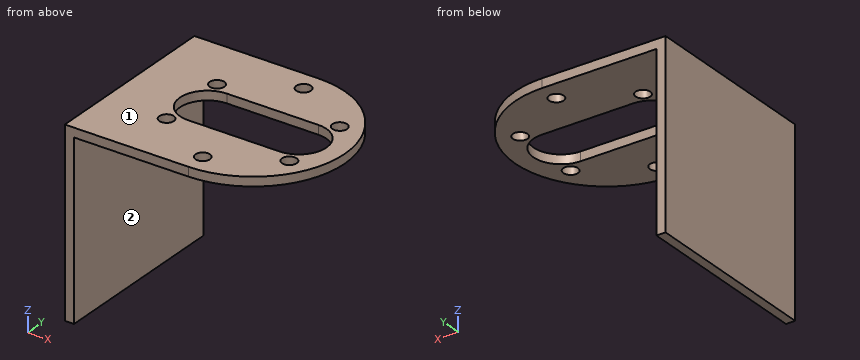
```python
from build123d import *

# Parameters (mm, degrees)
SKETCH_1_W               = 40
SKETCH_1_H               = 40
EXTRUDE_1_DEPTH          = 2
EXTRUDE_2_DEPTH          = 2
SKETCH_3_4_RX            = 1.6
SKETCH_3_4_RY            = 1.6
CUT_EXTRUDE_1_DEPTH      = 2
PATTERN_CIRCULAR_1_COUNT = 6
CUT_EXTRUDE_2_DEPTH      = 65.876806333


with BuildPart() as part:
    # 草图1 → 凸台-拉伸1 (new body)
    with BuildSketch(Plane(origin=(0, 0, 0), x_dir=(0, 0, -1), z_dir=(1, 0, 0))):
        Rectangle(SKETCH_1_W, SKETCH_1_H)
    extrude(amount=EXTRUDE_1_DEPTH)

    # 草图3 → 凸台-拉伸2 (add)
    with BuildSketch(Plane.XY.offset(20)):
        with BuildLine():
            Line((0, 20), (27, 20))
            ThreePointArc((27, 20), (47, 0), (27, -20))
            Line((27, -20), (0, -20))
            Line((0, -20), (0, 20))
        make_face()
    extrude(amount=-EXTRUDE_2_DEPTH)

    # 草图3<4> → 切除-拉伸1 (cut)
    with BuildSketch(Plane.XY.offset(20)):
        with Locations(Location((27.038693052, 15.512584913), (0, 0, 225))):
            Ellipse(SKETCH_3_4_RX, SKETCH_3_4_RY)
    cut_extrude_1 = extrude(amount=-CUT_EXTRUDE_1_DEPTH, mode=Mode.SUBTRACT)

    # 阵列(圆周)1: 切除-拉伸1 ×6 about axis
    pattern_circular_1_axis = Axis((27, 0, 0), (0, 0, 1))
    for i in range(1, PATTERN_CIRCULAR_1_COUNT):
        add(cut_extrude_1.rotate(pattern_circular_1_axis, i * 360 / PATTERN_CIRCULAR_1_COUNT), mode=Mode.SUBTRACT)

    # 草图3<5> → 切除-拉伸2 (cut, through all)
    with BuildSketch(Plane.XY.offset(20)):
        with BuildLine():
            Line((37, -6), (17, -6))
            ThreePointArc((17, -6), (11, 0), (17, 6))
            Line((17, 6), (37, 6))
            ThreePointArc((37, 6), (43, 0), (37, -6))
        make_face()
    extrude(amount=-CUT_EXTRUDE_2_DEPTH, mode=Mode.SUBTRACT)


solid = part.part
```
Read the model definition and answer for the solid it produces. Units are mm, in the model's axes. Face numbers are marked on the shaded views. A direction names the side the tool comes from. Give positions to 0.01 mm unless a question says otherwise; leave off trailing zeros. Write each loop counter-clockwise with the first axis right and the second up, starting at its lowest first coordinate (ties: lowest second). Pieces come first, ordered by that corner, then holes. Notation, with made-up numbers: M 51.5,4.25 L 110.5,4.25 A14 ccw 110.5,17.25 Z; hole C 43,81.5 d4. An arc over 180 degrees is marked long. Put each result on its own line as item: value. Start each with the question number.
1. Which of the six approach directions +Z, -Z, +X, -X, +Y, -Y give full straight-line access (tool end or side, diameter ignored) to the marked faces 1 and 2?
2. The part is cut by section A-A, the plane x = 22.5. Give the vertices of the cut face in (y, z), and give its area (3 significant figures).
3. The part is cut by section C-C, the plane z = 14. Give the vertices of the cut face in (x, y), and give its area (3 significant figures).
4. Each of these flat-tipped pins is pushed along its axis until it touches: pin 1 Ø1 at (x, z) = (31, 19.5) entering from +Y; pin 2 Ø10 at (x, y) = (38.5, 9) entering from -Z; pin 3 Ø11.5 at (y, z) = (-2, -1) entering from +X. Where does it stop, or does it pass through?
5. The part is cut by section B-B, the plane y = 0. Give the vertices of the cut face in (x, z), and give its area (3 significant figures).
6. The part is cut by section D-D, the plane x = 33. Give the vertices of the cut face in (y, z), and give its area (3 significant figures).
7. Consider line 1 along Z through (x, y) = (13, -11); line 2 along X through (y, z) = (15, 12). Determine where each line is inside the solid, lowest interval first.
Final values:
1. face 1: +Z, +X, -X, +Y, -Y
1. face 2: -Z, +X, +Y, -Y
2. outline: M -20,18 L -6,18 L -6,20 L -20,20 Z; M 6,18 L 20,18 L 20,20 L 6,20 Z
2. area: 56.0 mm²
3. outline: M 0,-20 L 2,-20 L 2,20 L 0,20 Z
3. area: 80.0 mm²
4. pin 1: stops at y = 19.69
4. pin 2: stops at z = 18
4. pin 3: stops at x = 2
5. outline: M 0,-20 L 2,-20 L 2,18 L 11,18 L 11,20 L 0,20 Z; M 43,18 L 47,18 L 47,20 L 43,20 Z
5. area: 106 mm²
6. outline: M -19.08,18 L -6,18 L -6,20 L -19.08,20 Z; M 6,18 L 19.08,18 L 19.08,20 L 6,20 Z
6. area: 52.3 mm²
7. line 1: z = 18 to 20
7. line 2: x = 0 to 2
